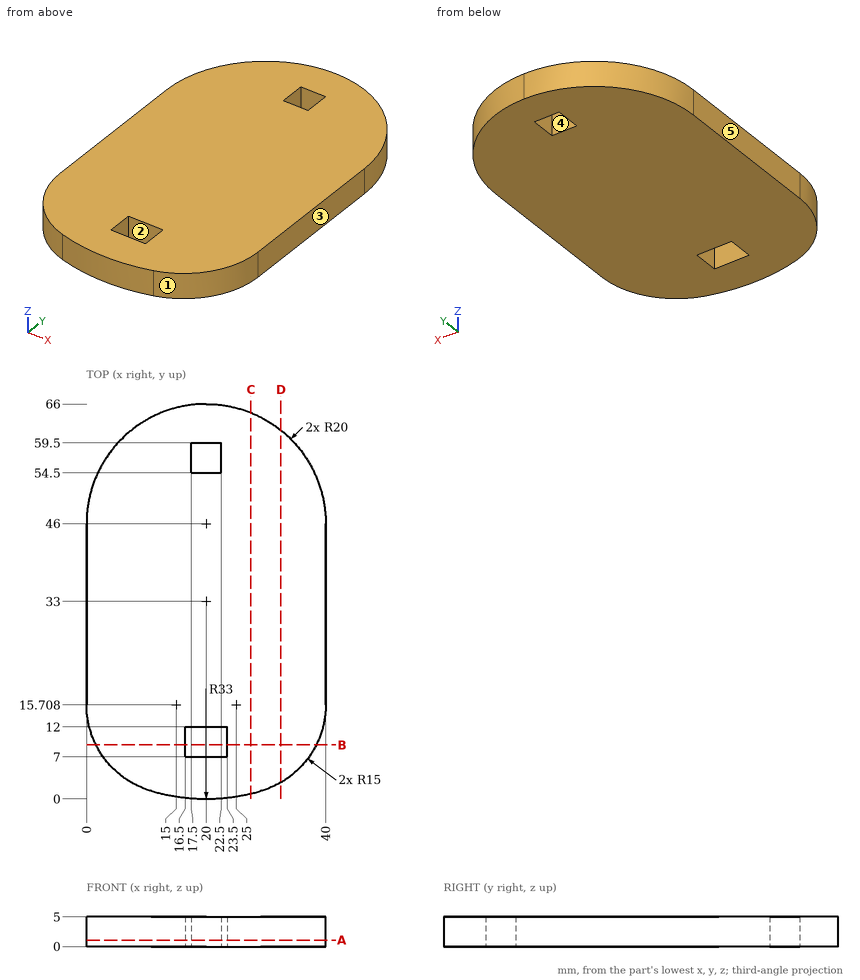
Source: three-view drawing plus pictorial views. Frame: mm from the lowest corner of the part. A direction names the side the tool comes from. Give positions to 0.01 mm unless a question says otherwise; leave off trailing zeros. Order: outer loops, then holes, each group sorted by start corner. A loop starts at its lowest first (then second) coordinate and runs counter-clockwise, first axis right, second up. Notation, with made-up numbers: (-13, 84.5) - (14, 84.5) arc R19 ccw to (14, 91.5) - close; hole circle Ø7 at (-32.5, -26.5). An arc over 180 degrees is marked (long way). Put each result on its own line as item: value.
Item 1: Ray query, L1, parallel to Y at x = 21, z = 4.7 (1 decimal); L2, parallel to Y at x = 8, z = 0.8; L3, parallel to Y at x = 9, z = 0.5 (1 decimal). Return the intervals inside material, ascending. Write a range as from..to.
Found:
L1: y = 0..7, 12..54.5, 59.5..66
L2: y = 2.44..62
L3: y = 2..62.7
Item 2: Section query D-D, the plane x = 32.5. Return loops of the section in (y, z).
Found:
outline: (2.72, 0) - (61.61, 0) - (61.61, 5) - (2.72, 5) - close
Item 3: Section query B-B, the plane y = 9. Return loops of the section in (x, z), then the cut area to 3 significant figures.
Found:
outline: (1.58, 0) - (16.5, 0) - (16.5, 5) - (1.58, 5) - close; (23.5, 0) - (38.42, 0) - (38.42, 5) - (23.5, 5) - close
area: 149 mm^2
Item 4: Access query for the marked faces 4 and 5. Directions: +Z, -Z, +X, -X, +Y, -Y. A direction counts if a zero-diameter tool reaches every point of the face in a straight line with its end or side. Return the directions, or none.
Found:
face 4: +Z, -Z
face 5: +Z, -Z, -X, +Y, -Y
Item 5: Draft query along Y for the marked faces 1, 2 and 3. Return one class per face: +Y half, -Y half, draft (parallel to the pull), parting line (faces both ways), or undercut.
Found:
face 1: -Y half
face 2: undercut
face 3: draft
Item 6: Section query A-A, the plane z = 1.1. Count the separate pieces of the cut face and the enclosed holes in it, then the cut area to 3 significant figures.
Found:
separate pieces: 1
enclosed holes: 2
area: 2,290 mm^2
Item 7: Contact query for flat-ended pins moving along their axis: pin 1 (2.5 mm diameter, centred on x = 20, z = 2, fed in from -Y); pin 2 (2 mm diameter, centred on x = 8, z = 1, fed in from +Y); pin 3 (1.5 mm diameter, centred on x = 21, z = 2, fed in from +Y). Output: stop coordinate, or through.
Found:
pin 1: stops at y = 0
pin 2: stops at y = 62.7
pin 3: stops at y = 66
Item 8: Section query C-C, the plane x = 27.5. Return loops of the section in (y, z).
Found:
outline: (0.86, 0) - (64.54, 0) - (64.54, 5) - (0.86, 5) - close
